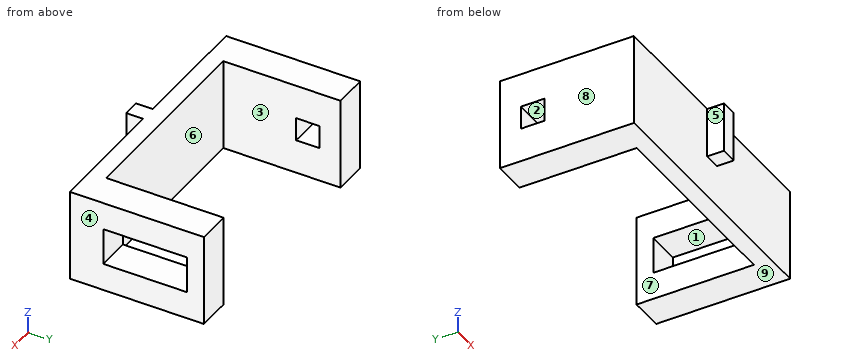
Autodesk Inventor part; units mm, degrees
ref_plane "YZ Plane" through (0, 0, 0) normal (1, 0, 0) x (0, 1, 0)
ref_plane "XZ Plane" through (0, 0, 0) normal (0, 1, 0) x (-1, 0, 0)
ref_plane "XY Plane" through (0, 0, 0) normal (0, 0, 1) x (1, 0, 0)
sketch "Boceto1" plane through (0, 0, 0) normal (0, 0, 1) x (1, 0, 0)
  line L0 (-80, 5) -> (80, 5)
  line L1 (80, 5) -> (80, -5)
  line L2 (80, -5) -> (-80, -5)
  line L3 (-80, -5) -> (-80, 5)
  line L4 (-80, 5) -> (80, -5) construction
  line L5 (80, 5) -> (-80, -5) construction
  point P0 (0, 0)
  dimension "d0" = 160
  dimension "d1" = 10
extrude "Extrusión1" add sketch "Boceto1" along normal blind 55
sketch "Boceto2" plane through (-80, 5, 0) normal (0, 1, 0) x (1, 0, 0)
  line L0 (0, 0) -> (0, -55)
  line L1 (0, -55) -> (160, -55)
  line L2 (0, 0) -> (20, 0)
  line L3 (20, 0) -> (20, -55)
  line L4 (20, -55) -> (0, -55)
  line L5 (0, -55) -> (0, 0)
  line L6 (160, 0) -> (160, -55)
  line L7 (160, 0) -> (140, 0)
  line L8 (140, 0) -> (140, -55)
  line L9 (140, -55) -> (160, -55)
  line L10 (160, -55) -> (160, 0)
  point P0 (80, 0)
  dimension "d4" = 20
  dimension "d5" = 20
extrude "Extrusión2" add sketch "Boceto2" along normal blind 70
sketch "Boceto3" plane through (-80, -5, 0) normal (-1, 0, 0) x (0, 0, 1)
  line L0 (0, 80) -> (55, 80)
  line L1 (20.5, 67.5) -> (34.5, 67.5)
  line L2 (34.5, 67.5) -> (34.5, 53.5)
  line L3 (34.5, 53.5) -> (20.5, 53.5)
  line L4 (20.5, 53.5) -> (20.5, 67.5)
  line L5 (20.5, 67.5) -> (34.5, 53.5) construction
  line L6 (34.5, 67.5) -> (20.5, 53.5) construction
  line L7 (0, 0) -> (0, 80)
  point P0 (0, 5)
  point P1 (27.5, 60.5)
  dimension "d10" = 14
  dimension "d11" = 14
  dimension "d12" = 20.5
  dimension "d13" = 12.5
extrude "Extrusión3" cut sketch "Boceto3" against normal blind 70
sketch "Boceto4" plane through (-80, -5, 0) normal (0, -1, 0) x (1, 0, 0)
  line L0 (140, 55) -> (20, 55)
  line L1 (75, 25) -> (85, 25)
  line L2 (85, 25) -> (85, 55)
  line L3 (85, 55) -> (75, 55)
  line L4 (75, 55) -> (75, 25)
  line L5 (75, 25) -> (85, 55) construction
  line L6 (85, 25) -> (75, 55) construction
  point P0 (80, 0)
  dimension "d17" = 10
  dimension "d30" = 30
extrude "Extrusión4" add sketch "Boceto4" along normal blind 10
sketch "Boceto5" plane through (80, -5, 55) normal (1, 0, 0) x (0, 0, -1)
  line L0 (0, 80) -> (55, 80)
  line L1 (55, 0) -> (55, 80)
  line L2 (16.5, 20) -> (16.5, 70)
  line L3 (16.5, 70) -> (38.5, 70)
  line L4 (38.5, 70) -> (38.5, 20)
  line L5 (38.5, 20) -> (16.5, 20)
  line L6 (16.5, 20) -> (38.5, 70) construction
  line L7 (16.5, 70) -> (38.5, 20) construction
  line L8 (0, 0) -> (0, 80)
  point P0 (55, 5)
  point P1 (27.5, 45)
  point P2 (16.5, 45)
  dimension "d26" = 50
  dimension "d27" = 22
  dimension "d28" = 16.5
  dimension "d29" = 10
extrude "Extrusión5" cut sketch "Boceto5" against normal blind 30
properties part number "camera_support"
Here's how the part is built. I have some questions about the finished solid (model axes, mm). Face numbers are marked on the shaded views. A direction names the side the tool comes from. Coordinates: 2 decimals unless noted, no trailing zeros. Order: outer loops, then holes, each group sorted by start corner. A loop starts at its lowest first (then second) coordinate and runs counter-clockwise, first axis right, second up. Notation, with made-up numbers: M 52,-12 L 71,-12 A33 ccw 71,24 Z; hole C 68.5,45.25 d10. An arc over 180 degrees is marked long. Answer as CSV lines item,"result". Start each with the question number.
1. On a 3-axis mill with a long thin cutter (end or side, diameter ignored), from which of +Z, -Z, +X, -X, +Y, -Y can I reach the whole of each face in a straight line? I mean the marked faces 1, 2, 3, 4 and 5. Say none if no direction works.
2. I want a section at B-B, the plane y = 21. Write out the boundary of the cut face in (x, z), and give its area (3 significant figures).
3. I want a section at C-C, the plane y = 67. Write out the boundary of the cut face in (x, z).
4. For pin 1 (3 mm diameter, centred on y = 24.5, z = 33, fed in from +X); pin 2 (5 mm diameter, centred on x = -12.5, z = 14, fed in from +Y); pin 3 (5 mm diameter, centred on y = -10.5, z = 46.5, fed in from -X); pin 4 (12 mm diameter, centred on x = 50, y = 56.5, fed in from +Z), each with a flat end and sliding along its axis, tell me the tip position at first contact or that it passes through.
5. We'd pull the mould along X, two halves only. Please class the marked faces 6, 7, 8 and 9: released by +X, released by -X, zero draft, split by the parting line, or undercut.
6. I want a section at D-D, the plane x = 2.5. Write out the boundary of the cut face in (y, z), and give its area (3 significant figures).
7. I want a section at A-A, the plane z = 23. Write out the boundary of the cut face in (x, y), and give its area (3 significant figures).
8. I need wall thicknesses on line 1 (X direction, y = 35.5, z = 13.5); line 2 (Z direction, x = 2, y = -9); line 3 (Y direction, x = -70, z = 44). Which ranges of each line are inside material? Lowest first, please. Write a range as [from, to].
Recorded:
1,face 1,"+X"
1,face 2,"+X, -X"
1,face 3,"+Z, -Z, +Y"
1,face 4,"+Z, -Z, +X, +Y, -Y"
1,face 5,"+Z, -Z, -X, -Y"
2,outline,"M -80,0 L -60,0 L -60,55 L -80,55 Z; M 60,0 L 80,0 L 80,16.5 L 60,16.5 Z; M 60,38.5 L 80,38.5 L 80,55 L 60,55 Z"
2,area,"1,760 mm2"
3,outline,"M -80,0 L -60,0 L -60,55 L -80,55 Z; M 60,0 L 80,0 L 80,55 L 60,55 Z"
4,pin 1,"stops at x = -60"
4,pin 2,"stops at y = 5"
4,pin 3,"stops at x = -5"
4,pin 4,"passes through"
5,face 6,"undercut"
5,face 7,"undercut"
5,face 8,"released by -X"
5,face 9,"zero draft"
6,outline,"M -15,25 L -5,25 L -5,0 L 5,0 L 5,55 L -15,55 Z"
6,area,"850 mm2"
7,outline,"M -80,-5 L 80,-5 L 80,15 L 60,15 L 60,5 L -60,5 L -60,48.5 L -80,48.5 Z; M -80,62.5 L -60,62.5 L -60,75 L -80,75 Z; M 60,65 L 80,65 L 80,75 L 60,75 Z"
7,area,"3,120 mm2"
8,line 1,"x = [-80, -60], [60, 80]"
8,line 2,"z = [25, 55]"
8,line 3,"y = [-5, 75]"
